The listing builds one solid part. Answer for the finished solid, in the listing's coordinates (mm). Coordinates: 2 decimals unless noted, no trailing zeros. Order: outer loops, then holes, each group sorted by start corner. A loop starts at its lowest first (then second) coordinate and runs counter-clockwise, first axis right, second up. Notation, with made-up numbers: (4, 2) -> (47, 2) arc R31 cw to (47, 40) -> close; hole circle Ø7 at (71.25, -13.75). An arc over 180 degrees is marked (long way). Answer in a Markdown table with one row per item.
```python
from build123d import *

# Parameters (mm, degrees)
EXTRUDE_START       = -4
EXTRUDE_1_OUTLINE_R = 4
EXTRUDE_1_DEPTH     = 4
EXTRUDE_START_2     = 6
SKETCH_2_R          = 5.9
SKETCH_2_R_2        = 2.1
EXTRUDE_2_DEPTH     = 6
SKETCH_3_R          = 1.7
CUT_EXTRUDE_1_DEPTH = 4


# Read off the part's stored shape, not the designer's step: 填料-伸長1
with BuildPart() as part:
    # 填料-伸長1 outline → 填料-伸長1 (new body)
    with BuildSketch(Plane(origin=(0, 20.156954032, 0), x_dir=(1, 0, 0), z_dir=(0, 1, 0)).offset(EXTRUDE_START)):
        with BuildLine():
            Line((-94.580009895, -253.67166291), (-53.224889363, -217.412126153))
            ThreePointArc((-53.224889363, -217.412126153), (-49.935495794, -207.73500968), (-59.959608209, -209.730971497))
            Line((-59.959608209, -209.730971497), (-101.314728741, -245.990508253))
            Line((-101.314728741, -245.990508253), (-94.580009895, -253.67166291))
        make_face()
        with Locations((-54.371772361, -211.624669079)):
            Circle(EXTRUDE_1_OUTLINE_R, mode=Mode.SUBTRACT)
    extrude(amount=EXTRUDE_1_DEPTH)

    # 草圖2 → 填料-伸長2 (add)
    with BuildSketch(Plane.XZ.offset(-16.156954032).offset(EXTRUDE_START_2)):
        with Locations(Location((-54.371772361, 211.624669079, 0), (0, 0, 198.721335886))):
            Circle(SKETCH_2_R)
        with Locations((-54.371772361, 211.624669079)):
            Circle(SKETCH_2_R_2, mode=Mode.SUBTRACT)
    extrude(amount=-EXTRUDE_2_DEPTH)

    # 草圖3 → 除料-伸長1 (cut)
    with BuildSketch(Plane.XZ.offset(-16.156954032)):
        with Locations((-73.169554421, 228.106276695)):
            Circle(SKETCH_3_R)
    extrude(amount=-CUT_EXTRUDE_1_DEPTH, mode=Mode.SUBTRACT)


solid = part.part
```
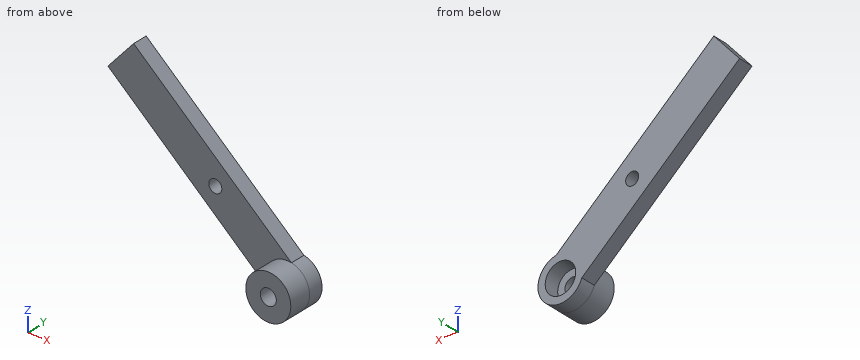
(1) A cutting plane is placed at D-D, the plane z = 227. Determine the outline of the cut face in (x, y).
Check values:
| item | result |
|---|---|
| outline | (-79.66, 16.16) -> (-74.46, 16.16) -> (-74.46, 20.16) -> (-79.66, 20.16) -> close; (-71.88, 16.16) -> (-64.16, 16.16) -> (-64.16, 20.16) -> (-71.88, 20.16) -> close |
(2) Find the intervals of material crossed by line 1 along Z through (x, y) = (-54, 11); line 2 along Y through (x, z) = (-56, 209.5); line 3 along Y through (x, z) = (-87, 244.5), in increasing order. Write a range as from..to.
Check values:
| item | result |
|---|---|
| line 1 | 205.74..209.56, 213.69..217.51 |
| line 2 | 10.16..16.16 |
| line 3 | 16.16..20.16 |
(3) A cutting plane is placed at A-A, the plane x = -74. Determine the outline of the cut face in (y, z), then the cut area to 3 significant figures.
Check values:
| item | result |
|---|---|
| outline | (16.16, 222.04) -> (20.16, 222.04) -> (20.16, 226.62) -> (16.16, 226.62) -> close; (16.16, 229.59) -> (20.16, 229.59) -> (20.16, 235.63) -> (16.16, 235.63) -> close |
| area | 42.5 mm² |
(4) Flat-ended cylindrical pins translate along their axes: pin 1 (3.5 mm diameter, centred on x = -54.37, z = 211.62, fed in from +Y); pin 2 (13 mm diameter, centred on x = -54.37, z = 211.62, fed in from -Y); pin 3 (13 mm diameter, centred on x = -77, z = 240, fed in from -Y); pin 4 (2.5 mm diameter, centred on x = -52.5, z = 210, fed in from +Y). Find the tip coordinate at first contact, or state that the pin passes through.
Check values:
| item | result |
|---|---|
| pin 1 | through |
| pin 2 | y = 10.16 |
| pin 3 | y = 16.16 |
| pin 4 | y = 16.16 |
(5) A cutting plane is placed at C-C, the plane y = 17. Determine the outline of the cut face in (x, z).
Check values:
| item | result |
|---|---|
| outline | (-101.31, 245.99) -> (-59.96, 209.73) arc R5.9 ccw (long way) to (-53.22, 217.41) -> (-94.58, 253.67) -> close; hole circle Ø3.4 at (-73.17, 228.11); hole circle Ø8 at (-54.37, 211.62) |
(6) A cutting plane is placed at B-B, the plane z = 212.5. Determine the outline of the cut face in (x, y), then the cut area to 3 significant figures.
Check values:
| item | result |
|---|---|
| outline | (-63.12, 16.16) -> (-60.21, 16.16) -> (-60.21, 10.16) -> (-56.28, 10.16) -> (-56.28, 16.16) -> (-58.27, 16.16) -> (-58.27, 20.16) -> (-63.12, 20.16) -> close; (-52.46, 10.16) -> (-48.54, 10.16) -> (-48.54, 20.16) -> (-50.47, 20.16) -> (-50.47, 16.16) -> (-52.46, 16.16) -> close |
| area | 74.2 mm² |
